Could you check a few things on this model? Use its own coordinates, in mm. A direction names the side the tool comes from. Coordinates: 2 decimals unless noted, no trailing zeros. Order: outer loops, then holes, each group sorted by start corner. A loop starts at its lowest first (then second) coordinate and runs counter-clockwise, first axis right, second up. Notation, with made-up numbers: (-19, 37) -> (28, 37) arc R29 cw to (28, 68) -> close; hole circle Ø1 at (24.5, 14.25). An arc over 180 degrees is marked (long way). Put each result on its own line as item: value. Start each with the question number.
Q1. If we section it at C-C (y = 28): Please give me the cut outline in (x, z).
Q2. For faces 5 (the face through (-4, 43, 0)), 6 (the face through (-2, 43, -43.6)), 7 (the face through (-4, 43, -40)), 8 (the face through (-2, 79, 2)), 9 (the face through (-13.597, 42.891, -19.701)), which set-ups out of +Z, -Z, +X, -X, +Y, -Y let a thin tool reach every point of the face, with its end or its side?
Q3. We'd pull the mould along Z, two halves only. Please class faces 1 (the face through (-17.497, 42.905, -19.682)), 2 (the face through (0, 43, -39)), 3 (the face through (-2, 12, -39)), 4 (the face through (-0.986, 12.934, -41.817)): +Z half, -Z half, draft (parallel to the pull), parting line (faces both ways), or undercut.
Q4. If we section it at B-B (z = 0.5): Please give me the cut outline in (x, y), and give its area (3 significant figures).
Q5. If we section it at D-D (z = -20): Please give me the cut outline in (x, y).
Q6. Please list where these lines run through material, in increasing order: line 1 along Z through (x, y) = (-1.4, 79); line 2 along X through (y, z) = (29.5, -40.5); line 3 along Z through (x, y) = (-1, 13).
Q7. If we section it at A-A (y = 13): Count the separate pieces of the cut face and the enclosed holes in it, and give its area (3 significant figures).
Q8. Will these pins go through, and if not, where does the flat tip stop? pin 1 (1.5 mm diameter, centred on y = 13.5, z = -0.5, fed in from -X); pin 2 (5.5 mm diameter, centred on y = 79, z = -40, fed in from -X); pin 3 (2 mm diameter, centred on x = -11.5, y = 13.5, fed in from -Z).
Autodesk Inventor part; units mm, degrees
ref_plane "YZ Plane" through (0, 0, 0) normal (1, 0, 0) x (0, 1, 0)
ref_plane "XZ Plane" through (0, 0, 0) normal (0, 1, 0) x (-1, 0, 0)
ref_plane "XY Plane" through (0, 0, 0) normal (0, 0, 1) x (1, 0, 0)
sketch "スケッチ1" plane through (0, 0, 0) normal (0, 1, 0) x (-1, 0, 0)
  line L0 (0, 0) -> (20, 0)
  line L1 (20, 0) -> (20, -40)
  line L2 (20, -40) -> (0, -40)
  line L3 (0, -40) -> (0, 0)
  circle A0 centre (0, -20) radius 13.6
  circle A1 centre (0, -20) radius 17.5
  line L4 (0, -6.4) -> (4, -6.4)
  line L5 (4, -6.4) -> (4, 3.6)
  line L6 (4, 3.6) -> (0, 3.6)
  line L7 (0, 3.6) -> (0, -6.4)
  line L8 (0, -33.6) -> (4, -33.6)
  line L9 (4, -33.6) -> (4, -43.6)
  line L10 (4, -43.6) -> (0, -43.6)
  line L11 (0, -43.6) -> (0, -33.6)
  point P0 (0, -6.4)
  point P1 (0, -33.6)
  point P2 (4, -37.0367)
  point P3 (4, -2.9633)
  dimension "d0" = 20
  dimension "d1" = 40
  dimension "d2" = 27.2
  dimension "d3" = 35
  dimension "d4" = 4
  dimension "d5" = 10
  dimension "d6" = 4
  dimension "d7" = 10
extrude "押し出し1" add sketch "スケッチ1" along normal blind 87 contours L7 L6 L5 L0 | L0 L5 A1 L3 | A1 L5 L4 L3 | A1 L9 L8 A0 L4 L5 | A1 L9 L2 L3 | L3 L8 L9 A1 | L2 L9 L10 L11
sketch "スケッチ2" plane through (-4, 0, -43.6) normal (-1, 0, 0) x (0, 0, 1)
  line L0 (0, 87) -> (6.5633, 87)
  line L1 (40.6367, 87) -> (47.2, 87)
  line L2 (40.6367, 0) -> (47.2, 0)
  line L3 (0, 0) -> (6.5633, 0)
  point P0 (43.6, 0)
  point P1 (3.2816, 13)
  point P2 (3.2816, 79)
  point P3 (43.9184, 79)
  point P4 (43.9184, 13)
  point P5 (3.2816, 87)
  point P6 (43.9184, 87)
  point P7 (43.9184, 0)
  point P8 (3.2816, 0)
  dimension "d10" = 0
  dimension "d11" = 8
  dimension "d12" = 0
  dimension "d13" = 8
  dimension "d14" = 0
  dimension "d15" = 0
  dimension "d16" = 13
  dimension "d17" = 13
hole "穴1" at (-4, 13, -40.3184) at (-4, 79, -40.3184) at (-4, 79, 0.3184) at (-4, 13, 0.3184) direction (1, 0, 0) diameter 3 end through all
fillet "フィレット1" radius 1 14 edges at (-4, 87, 0.3184) (-17.5, 87, -20) (-4, 87, -40.3184) (-2, 87, -43.6) (-2, 87, 3.6) (-4, 43.5, 3.6) (-4, 0, 0.3184) (-17.5, 0, -20) (-4, 0, -40.3184) (-2, 0, -43.6) (-2, 0, 3.6) (-4, 43.5, -43.6) (-4, 43.5, -37.0367) (-4, 43.5, -2.9633)
sketch "スケッチ5" plane through (-4, 1, -37.8115) normal (-1, 0, 0) x (0, 0, 1)
  circle A0 centre (-2.5068, 12) radius 1.5
  circle A1 centre (-2.5068, 12) radius 2.5
  circle A2 centre (38.1299, 12) radius 1.5
  circle A3 centre (38.1299, 12) radius 2.5
  circle A4 centre (-2.5068, 78) radius 1.5
  circle A5 centre (-2.5068, 78) radius 2.5
  circle A6 centre (38.1299, 78) radius 1.5
  circle A7 centre (38.1299, 78) radius 2.5
  point P0 (37.8115, -1)
  dimension "d36" = 5
  dimension "d37" = 5
  dimension "d38" = 5
  dimension "d39" = 5
extrude "押し出し4" cut sketch "スケッチ5" against normal blind 2
properties part number "arm-2-2_3D プリント"
The answers:
1. outline: (-4.73, -36.85) arc R1 cw to (-4, -37.81) -> (-4, -42.6) arc R1 ccw to (-3, -43.6) -> (0, -43.6) -> (0, -33.6) arc R13.6 cw to (0, -6.4) -> (0, 3.6) -> (-3, 3.6) arc R1 ccw to (-4, 2.6) -> (-4, -2.19) arc R1 cw to (-4.73, -3.15) arc R17.5 ccw to start
2. face 5: +Z, -X, +Y, -Y
2. face 6: -Z, +X, -X, +Y, -Y
2. face 7: -Z, -X, +Y, -Y
2. face 8: -X
2. face 9: +X, +Y, -Y
3. face 1: parting line
3. face 2: draft
3. face 3: undercut
3. face 4: undercut
4. outline: (-4, 1) arc R1 ccw to (-3, 0) -> (0, 0) -> (0, 11.51) -> (-2, 11.51) -> (-2, 10.51) -> (-4, 10.51) -> close; (-4, 15.49) -> (-2, 15.49) -> (-2, 14.49) -> (0, 14.49) -> (0, 77.51) -> (-2, 77.51) -> (-2, 76.51) -> (-4, 76.51) -> close; (-4, 81.49) -> (-2, 81.49) -> (-2, 80.49) -> (0, 80.49) -> (0, 87) -> (-3, 87) arc R1 ccw to (-4, 86) -> close
4. area: 316 mm^2
5. outline: (-17.5, 1) arc R1 ccw to (-16.5, 0) -> (-13.6, 0) -> (-13.6, 87) -> (-16.5, 87) arc R1 ccw to (-17.5, 86) -> close
6. line 1: -43.6 to -41.82, -38.82 to -33.53, -6.47 to -1.18, 1.82 to 3.6
6. line 2: -4 to 0
6. line 3: -43.6 to -41.82, -38.82 to -33.56, -6.44 to -1.18, 1.82 to 3.6
7. separate pieces: 3
7. enclosed holes: 0
7. area: 208 mm^2
8. pin 1: x = -2
8. pin 2: x = -4.17
8. pin 3: z = -34
